Read the model definition and answer for the solid it produces. Units are mm, in the model's axes. A direction names the side the tool comes from. Coordinates: 2 decimals unless noted, no trailing zeros. Write each loop counter-clockwise with the first axis right and the second up, starting at its lowest first coordinate (ties: lowest second). Pieces come first, ordered by that corner, then holes. Notation, with made-up numbers: (85, 79.5) -> (124, 79.5) arc R16 cw to (124, 83.5) -> close; hole circle Ø1 at (28, 52.25). An arc over 180 degrees is marked (long way). Return JSON: item names as keys, results as strings.
from build123d import *

# Parameters (mm, degrees)
SKICA2_W                = 72.4
SKICA2_H                = 47.7
P_IDAT_VYSUNUT_M1_DEPTH = 1.2
SKICA3_W                = 70
SKICA3_H                = 46.5
P_IDAT_VYSUNUT_M2_DEPTH = 1
SKICA4_W                = 70
SKICA4_H                = 7
P_IDAT_VYSUNUT_M3_DEPTH = 7
ZKOSEN_2_SIZE           = 7


with BuildPart() as part:
    # Skica2 → Přidat vysunutím1 (new body)
    with BuildSketch(Plane(origin=(0, 0, 0), x_dir=(1, 0, 0), z_dir=(0, 1, 0))):
        with Locations((36.2, 23.85)):
            Rectangle(SKICA2_W, SKICA2_H)
    extrude(amount=P_IDAT_VYSUNUT_M1_DEPTH)

    # Skica3 → Přidat vysunutím2 (add)
    with BuildSketch(Plane(origin=(0, 1.2, 0), x_dir=(1, 0, 0), z_dir=(0, 1, 0))):
        with Locations((36.2, 24.45)):
            Rectangle(SKICA3_W, SKICA3_H)
    extrude(amount=P_IDAT_VYSUNUT_M2_DEPTH)

    # Skica4 → Přidat vysunutím3 (add)
    with BuildSketch(Plane(origin=(0, 2.2, 0), x_dir=(1, 0, 0), z_dir=(0, 1, 0))):
        with Locations((36.2, 44.2)):
            Rectangle(SKICA4_W, SKICA4_H)
    extrude(amount=P_IDAT_VYSUNUT_M3_DEPTH)

    # Zkosení2
    zkosen_2_edges = [part.edges().sort_by_distance(p)[0] for p in [
        (36.2, 9.2, -40.7),
    ]]
    chamfer(zkosen_2_edges, length=ZKOSEN_2_SIZE - 0.0001)  # a hair under: the kernel refuses the full size


solid = part.part
1. A tool of negligible diameter and unlimited length cuts with its end or side. For faces 1 (the face through (36, 5, -47.7)), 2 (the face through (71.2, 2, -31)), 3 (the face through (36, 0, -24)), 4 (the face through (1.2, 2, -31)), 5 (the face through (36, 2.2, -21)), from which of +Z, -Z, +X, -X, +Y, -Y can it reach the whole face along a straight path? Write none if from no direction.
Taken from the geometry:
{"face 1": "-Z, +X, -X, +Y, -Y", "face 2": "+Z, -Z, +X, +Y", "face 3": "+Z, -Z, +X, -X, -Y", "face 4": "+Z, -Z, -X, +Y", "face 5": "+Z, +X, -X, +Y"}
2. The part is cut by section A-A (z = -22). Determine the outline of the cut face in (x, y), then the cut area to 3 significant figures.
Taken from the geometry:
{"outline": "(0, 0) -> (72.4, 0) -> (72.4, 1.2) -> (71.2, 1.2) -> (71.2, 2.2) -> (1.2, 2.2) -> (1.2, 1.2) -> (0, 1.2) -> close", "area": "157 mm2"}
3. Flat-ended cylindrical pins translate along their axes: pin 1 Ø24 at (x, z) = (30.5, -29.5) entering from +Y; pin 2 Ø1 at (x, y) = (49.5, 5.5) entering from +Z. Find the tip coordinate at first contact, or state that the pin passes through.
Taken from the geometry:
{"pin 1": "stops at y = 3", "pin 2": "stops at z = -43.5"}
4. The part is cut by section C-C (y = 8.25). Determine the outline of the cut face in (x, z).
Taken from the geometry:
{"outline": "(1.2, -47.7) -> (71.2, -47.7) -> (71.2, -46.75) -> (1.2, -46.75) -> close"}
5. Consider L1, parallel to Y at x = 41, z = -15.5; L2, parallel to X at y = 1.75, z = -6; L3, parallel to Z at x = 61.5, y = 2. Determine where each line is inside the solid, lowest interval first.
Taken from the geometry:
{"L1": "y = 0 to 2.2", "L2": "x = 1.2 to 71.2", "L3": "z = -47.7 to -1.2"}
